```python
from build123d import *


with BuildPart() as part:
    # Sketch1 → Revolve1 (revolve)
    with BuildSketch(Plane(origin=(0, 0, 0), x_dir=(1, 0, 0), z_dir=(0, 1, 0))):
        with BuildLine():
            Line((0, 0), (0, 13.25))
            ThreePointArc((0, 13.25), (0.585786438, 14.664213562), (2, 15.25))
            Line((2, 15.25), (19, 15.25))
            Line((19, 15.25), (19, 16.3))
            ThreePointArc((19, 16.3), (19.058578644, 16.441421356), (19.2, 16.5))
            Line((19.2, 16.5), (59.5, 16.5))
            ThreePointArc((59.5, 16.5), (59.853553391, 16.353553391), (60, 16))
            Line((60, 16), (60, 15.6))
            ThreePointArc((60, 15.6), (59.853553391, 15.246446609), (59.5, 15.1))
            Line((59.5, 15.1), (32, 15.1))
            ThreePointArc((32, 15.1), (30.585786438, 14.514213562), (30, 13.1))
            Line((30, 13.1), (30, 0))
            Line((30, 0), (0, 0))
        make_face()
    revolve(axis=Axis((30, 0, 0), (-1, 0, 0)))


solid = part.part
```
For this review, take the finished solid that the model builds, in its own axes (mm). A direction names the side the tool comes from. Round coordinates to 2 decimals unless told otherwise and drop trailing zeros. Write each loop counter-clockwise with the first axis right and the second up, starting at its lowest first coordinate (ties: lowest second). Pieces come first, ordered by that corner, then holes. Notation, with made-up numbers: (68, 33) - (75, 33) arc R21 cw to (75, 66) - close; hole circle Ø7 at (55, -21). An arc over 180 degrees is marked (long way). Answer as a JSON object with one key per item and string values.
1. Draft analysis for pull direction Y (two halves, no side actions). For faces 1 (the face through (39.63, 6.32, -15.24)), 2 (the face through (45.56, 14.74, 3.27)), 3 (the face through (30, 0, 0)), 4 (the face through (19, 11, 11)), state which applies: +Y half, -Y half, draft (parallel to the pull), parting line (faces both ways), or undercut.
Response values:
{"face 1": "parting line", "face 2": "undercut", "face 3": "undercut", "face 4": "draft"}
2. We need section C-C on x = 52. Give the boundary of the cut face in (y, z).
Response values:
{"outline": "circle Ø33 at (0, 0); hole circle Ø30.2 at (0, 0)"}
3. Tool access review of faces 5 (the face through (10.62, 9.28, 12.1)), 6 (the face through (0, 0, 0)): name each direction out of +Z, -Z, +X, -X, +Y, -Y from which nothing blocks a thin tool from reaching the whole face with its end or side.
Response values:
{"face 5": "-X", "face 6": "+Z, -Z, -X, +Y, -Y"}
4. For pin 1 Ø8 at (y, z) = (-4.5, 2.5) entering from +X; pin 2 Ø4 at (x, y) = (9, -7.5) entering from +Z; pin 3 Ø6 at (x, y) = (46, 3.5) entering from +Z, all flat-tipped, find the tip position at first contact; note any pin that passes through.
Response values:
{"pin 1": "stops at x = 30", "pin 2": "stops at z = 14.22", "pin 3": "stops at z = 16.49"}
5. We need section A-A on y = 0. Give the boundary of the cut face in (x, z).
Response values:
{"outline": "(0, -13.25) arc R2 ccw to (2, -15.25) - (19, -15.25) - (19, -16.3) arc R0.2 ccw to (19.2, -16.5) - (59.5, -16.5) arc R0.5 ccw to (60, -16) - (60, -15.6) arc R0.5 ccw to (59.5, -15.1) - (32, -15.1) arc R2 cw to (30, -13.1) - (30, 13.1) arc R2 cw to (32, 15.1) - (59.5, 15.1) arc R0.5 ccw to (60, 15.6) - (60, 16) arc R0.5 ccw to (59.5, 16.5) - (19.2, 16.5) arc R0.2 ccw to (19, 16.3) - (19, 15.25) - (2, 15.25) arc R2 ccw to (0, 13.25) - close"}
6. To check wall thickness, follow line 1 along Z through (x, y) = (42, 0); line 2 along X through (y, z) = (10.5, 12); line 3 along X through (y, z) = (-1.5, -12). State the ranges of each line that lie inside material, in increasing order.
Response values:
{"line 1": "z = -16.5 to -15.1, 15.1 to 16.5", "line 2": "x = 19 to 60", "line 3": "x = 0 to 30"}
